Geometry: see drawing. Coordinates: mm, zero at the bounding-box minimum. Coordinates: 2 decimals unless noted, no trailing zeros. Loops run counter-clockwise (first coordinate to the right, second up) from the corner with the lowest first, then second, coordinate; pieces in that order, holes last. Notation, with made-up numbers: (10, 58) - (53, 58) arc R10 cw to (53, 75) - close; hole circle Ø4 at (-7, 16). An arc over 180 degrees is marked (long way). Answer in a Markdown table with one row per item.
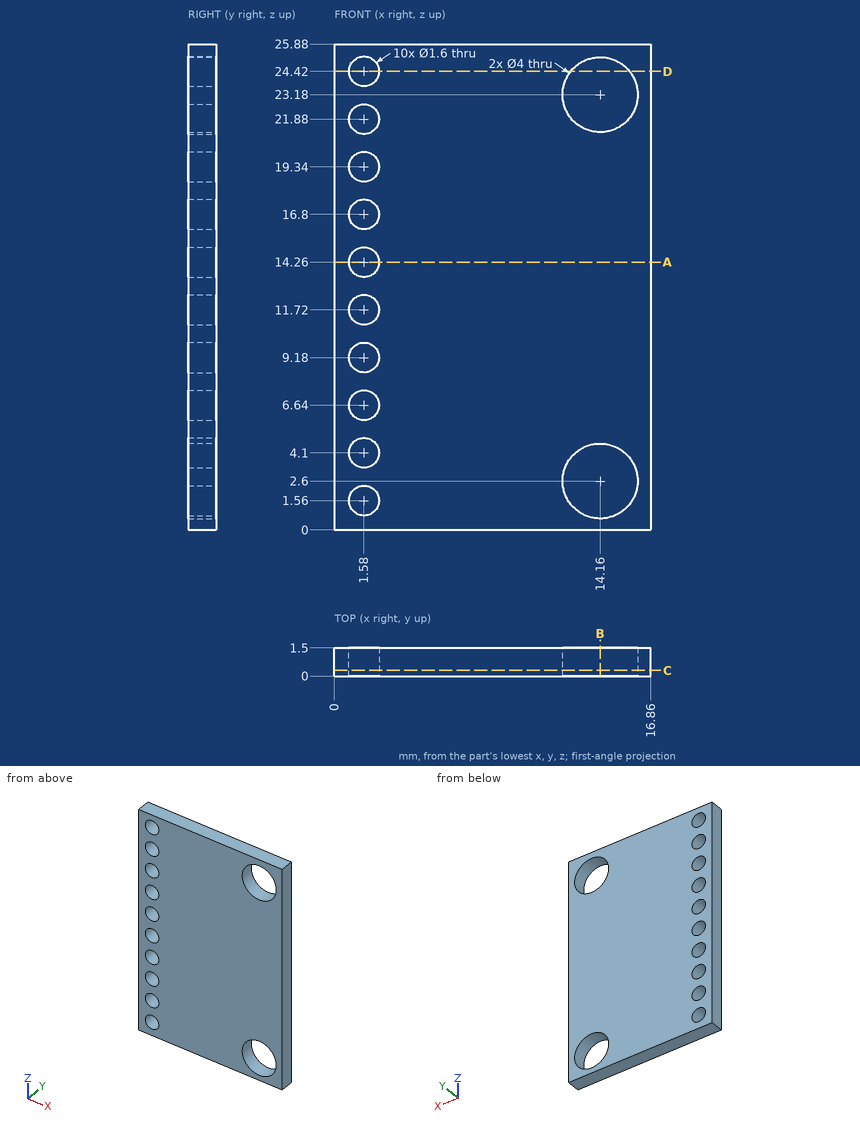
(1) First-contact query: pin 1 Ø1.8 at (x, z) = (1.58, 1.56) entering from +Y. Flat tip, straight axial feed; report the tip coordinate or a pass-through.
Verdict:
| item | result |
|---|---|
| pin 1 | stops at y = 1.5 |
(2) Cut plane A-A on z = 14.26. Output: boundary loops of the cut face in (x, y).
Verdict:
| item | result |
|---|---|
| outline | (0, 0) - (0.78, 0) - (0.78, 1.5) - (0, 1.5) - close; (2.38, 0) - (16.86, 0) - (16.86, 1.5) - (2.38, 1.5) - close |
(3) Cut plane B-B on x = 14.16. Output: boundary loops of the cut face in (y, z).
Verdict:
| item | result |
|---|---|
| outline | (0, 0) - (1.5, 0) - (1.5, 0.6) - (0, 0.6) - close; (0, 4.6) - (1.5, 4.6) - (1.5, 21.18) - (0, 21.18) - close; (0, 25.18) - (1.5, 25.18) - (1.5, 25.88) - (0, 25.88) - close |
(4) Cut plane D-D on z = 24.42. Output: boundary loops of the cut face in (x, y), then the cut area to 3 significant figures.
Verdict:
| item | result |
|---|---|
| outline | (0, 0) - (0.78, 0) - (0.78, 1.5) - (0, 1.5) - close; (2.38, 0) - (12.59, 0) - (12.59, 1.5) - (2.38, 1.5) - close; (15.73, 0) - (16.86, 0) - (16.86, 1.5) - (15.73, 1.5) - close |
| area | 18.2 mm² |
(5) Cut plane C-C on y = 0.3. State how many separate pieces and enclosed holes the cut face has, then the cut area to 3 significant figures.
Verdict:
| item | result |
|---|---|
| separate pieces | 1 |
| enclosed holes | 12 |
| area | 391 mm² |
(6) Ray query, probe 1 along Z at (x, y) = (14.16, 0.65); probe 2 along X at (y, z) = (0.8, 2.6); probe 3 along Z at (x, y) = (13, 1.15). Return the intervals inside material, ascending.
Verdict:
| item | result |
|---|---|
| probe 1 | z = 0 to 0.6, 4.6 to 21.18, 25.18 to 25.88 |
| probe 2 | x = 0 to 12.16, 16.16 to 16.86 |
| probe 3 | z = 0 to 0.97, 4.23 to 21.55, 24.81 to 25.88 |
